```python
from build123d import *

# Parameters (mm, degrees)
BOSS_EXTRUDE2_DEPTH = 1.5
CUTPLANE1_SKETCH_W  = 123.196195192
CUTPLANE1_SKETCH_H  = 53.525097373
CUT_EXTRUDE6_DEPTH  = 111
CUTPLANE2_SKETCH_W  = 123.196195192
CUTPLANE2_SKETCH_H  = 53.525097373
CUT_EXTRUDE7_DEPTH  = 111


with BuildPart() as part:
    # Sketch1 → Revolve1 (revolve)
    with BuildSketch(Plane.XY, mode=Mode.PRIVATE) as revolve1_sk:
        with BuildLine():
            Line((0, 0), (-48, 0))
            Line((-48, 0), (-48, -2))
            Line((-48, -2), (-46, -2))
            Line((-46, -2), (-42.202855897, -27.901871877))
            Line((-42.202855897, -27.901871877), (-40.181479372, -27.901871877))
            Line((-40.181479372, -27.901871877), (-43.810762695, -3.145046985))
            ThreePointArc((-43.810762695, -3.145046985), (-43.577990749, -2.346183124), (-42.821337927, -2))
            Line((-42.821337927, -2), (0, -2))
            Line((0, -2), (0, 0))
        make_face()
    revolve(revolve1_sk.sketch.rotate(Axis((0, 0, 0), (0, -1, 0)), 270), axis=Axis((0, 0, 0), (0, -1, 0)))

    # Sketch13 → Boss-Extrude2 (add, symmetric)
    with BuildSketch(Plane(origin=(0, 0, 0), x_dir=(0, 0, -1), z_dir=(1, 0, 0))):
        Polygon((-45.341508105, -0.931589376), (45.341508105, -0.931589376), (41.320088317, -28.8804569), (-41.722230296, -28.8804569), align=None)
    extrude(amount=BOSS_EXTRUDE2_DEPTH, both=True)

    # CutPlane1 Sketch → Cut-Extrude6 (cut)
    with BuildSketch(Plane(origin=(8, 0, 0), x_dir=(0, 0, -1), z_dir=(1, 0, 0))):
        with Locations((0.221178088, -12.173153045)):
            Rectangle(CUTPLANE1_SKETCH_W, CUTPLANE1_SKETCH_H)
    extrude(amount=CUT_EXTRUDE6_DEPTH, mode=Mode.SUBTRACT)

    # CutPlane2 Sketch → Cut-Extrude7 (cut)
    with BuildSketch(Plane(origin=(-8, 0, 0), x_dir=(0, 0, -1), z_dir=(1, 0, 0))):
        with Locations((0.221178088, -12.173153045)):
            Rectangle(CUTPLANE2_SKETCH_W, CUTPLANE2_SKETCH_H)
    extrude(amount=-CUT_EXTRUDE7_DEPTH, mode=Mode.SUBTRACT)


solid = part.part
```
Read the model definition and answer for the solid it produces. Units are mm, in the model's axes. Give positions to 0.01 mm unless a question says otherwise; leave off trailing zeros. Loops run counter-clockwise (first coordinate to the right, second up) from the corner with the lowest first, then second, coordinate; pieces in that order, holes last.
Item 1: The part is cut by section A-A (z = 29). Write down the section's boundary in (x, y).
Item 2: Each of these flat-tipped pins is pushed along its axis until it touches: pin 1 Ø1.5 at (y, z) = (-4.5, -33.5) entering from -X; pin 2 Ø2 at (x, y) = (2, -15) entering from +Z; pin 3 Ø2 at (x, z) = (5.5, 11) entering from -Y. Where does it stop, or does it pass through?
Item 3: Find the intervals of material crossed by line 1 along X through (y, z) = (-18.5, -35); line 2 along Z through (x, y) = (7, -17); line 3 along Z through (x, y) = (6, -24.5), in increasing order.
Item 4: The mould has two halves that part along X. Classify faces 1 (the conical face through (4.968, -15.35, 41.727)), 2 (the conical face through (-4.968, -15.35, -41.727)), 3 (the flat face through (0, -2, -47)), 4 (the flat face through (-8, -1, 0)): released by +X, released by -X, zero draft, split by the parting line, or undercut.
Item 5: The part is cut by section B-B (y = -8.75). Write down the section's boundary in (x, z), and give its area (3 significant figures).
Item 6: The part is cut by section C-C (y = -19.5). Write down the section's boundary in (x, z).
Taken from the geometry:
1. outline: (-8, -2) - (-1.5, -2) - (-1.5, -28.88) - (1.5, -28.88) - (1.5, -2) - (8, -2) - (8, 0) - (-8, 0) - close
2. pin 1: stops at x = -1.5
2. pin 2: stops at z = 44.2
2. pin 3: stops at y = -2
3. line 1: x = -1.5 to 1.5
3. line 2: z = -43.24 to -41.19, 41.19 to 43.24
3. line 3: z = -42.28 to -40.24, 40.24 to 42.28
4. face 1: undercut
4. face 2: undercut
4. face 3: zero draft
4. face 4: released by -X
5. outline: (-8, -44.29) arc R45.01 ccw to (8, -44.29) - (8, -42.24) arc R42.99 cw to (1.5, -42.96) - (1.5, 42.96) arc R42.99 cw to (8, 42.24) - (8, 44.29) arc R45.01 ccw to (-8, 44.29) - (-8, 42.24) arc R42.99 cw to (-1.5, 42.96) - (-1.5, -42.96) arc R42.99 cw to (-8, -42.24) - close
5. area: 323 mm2
6. outline: (-8, -42.69) arc R43.43 ccw to (8, -42.69) - (8, -40.63) arc R41.41 cw to (1.5, -41.39) - (1.5, 41.39) arc R41.41 cw to (8, 40.63) - (8, 42.69) arc R43.43 ccw to (-8, 42.69) - (-8, 40.63) arc R41.41 cw to (-1.5, 41.39) - (-1.5, -41.39) arc R41.41 cw to (-8, -40.63) - close
